Autodesk Inventor part; units mm, degrees
ref_plane "YZ Plane" through (0, 0, 0) normal (1, 0, 0) x (0, 1, 0)
ref_plane "XZ Plane" through (0, 0, 0) normal (0, 1, 0) x (-1, 0, 0)
ref_plane "XY Plane" through (0, 0, 0) normal (0, 0, 1) x (1, 0, 0)
sketch "Sketch1" plane through (0, 0, 0) normal (0, 1, 0) x (-1, 0, 0)
  line L0 (65, 81) -> (-65, 81)
  line L1 (-65, 81) -> (-65, -81)
  line L2 (-65, -81) -> (65, -81)
  line L3 (65, -81) -> (65, 81)
  point P0 (0, 0)
  point P1 (65, 0)
  point P2 (0, -81)
  dimension "d0" = 162
  dimension "d1" = 130
extrude "Extrusion1" add sketch "Sketch1" along normal blind 4
sketch "Sketch2" plane through (0, 4, 0) normal (0, 1, 0) x (1, 0, 0)
  circle A0 centre (-30, 0) radius 6
  circle A1 centre (30, 0) radius 6
  line L0 (-30, 6) -> (30, 6)
  line L1 (-30, -6) -> (30, -6)
  point P0 (0, 0)
  dimension "d4" = 12
  dimension "d5" = 12
  dimension "d6" = 30
  dimension "d7" = 30
extrude "Extrusion2" cut sketch "Sketch2" against normal through all
sketch "Sketch3" plane through (65, 0, 81) normal (1, 0, 0) x (0, 0, -1)
  line L0 (0, 4) -> (162, 4)
  line L1 (0, 0) -> (162, 0)
  line L2 (51, 4) -> (111, 4)
  line L3 (111, 4) -> (111, 0)
  line L4 (111, 0) -> (51, 0)
  line L5 (51, 0) -> (51, 4)
  point P0 (81, 0)
  point P1 (81, 0)
  dimension "d10" = 60
  dimension "d11" = 30
extrude "Extrusion3" add sketch "Sketch3" along normal blind 12
sketch "Sketch4" plane through (0, 4, 0) normal (0, 1, 0) x (1, 0, 0)
  line L0 (-65, -81) -> (65, -81)
  line L1 (-65, -81) -> (-55, -81)
  line L2 (-55, -81) -> (-55, -61)
  line L3 (-55, -61) -> (-65, -61)
  line L4 (-65, -61) -> (-65, -81)
  point P0 (0, 0)
  dimension "d14" = 20
  dimension "d15" = 10
extrude "Extrusion4" cut sketch "Sketch4" against normal blind 4
mirror "Mirror1" about plane through (0, 0, 0) normal (0, 0, 1) of "Extrusion4"
sketch "Sketch5" plane through (65, 0, 81) normal (0, 0, 1) x (1, 0, 0)
  line L0 (-35, 4) -> (-95, 4)
  line L1 (-80, 4) -> (-30, 4)
  line L2 (-30, 4) -> (-30, 0)
  line L3 (-30, 0) -> (-80, 0)
  line L4 (-80, 0) -> (-80, 4)
  line L5 (0, 0) -> (0, 4)
  point P0 (-65, 0)
  point P1 (-30, 2)
  point P2 (-80, 2)
  point P3 (0, 2)
  point P4 (-55, 0)
  dimension "d18" = 50
  dimension "d19" = 55
extrude "Extrusion5" add sketch "Sketch5" along normal blind 12
sketch "Sketch6" plane through (0, 4, 0) normal (0, 1, 0) x (1, 0, 0)
  line L0 (0, -85) -> (20, -85)
  line L1 (20, -85) -> (20, -89)
  line L2 (20, -89) -> (0, -89)
  line L3 (0, -89) -> (0, -85)
  line L4 (35, -81) -> (65, -81)
  line L5 (35, -81) -> (35, -93)
  point P0 (0, 0)
  point P1 (20, -87)
  dimension "d22" = 20
  dimension "d23" = 4
  dimension "d24" = 4
  dimension "d25" = 15
extrude "Extrusion6" cut sketch "Sketch6" against normal blind 12
mirror "Mirror2" about plane through (0, 0, 0) normal (0, 0, 1) of "Extrusion5", "Extrusion6"
sketch "Sketch7" plane through (0, 4, 0) normal (0, 1, 0) x (1, 0, 0)
  line L0 (69, 15) -> (73, 15)
  line L1 (73, 15) -> (73, -15)
  line L2 (73, -15) -> (69, -15)
  line L3 (69, -15) -> (69, 15)
  line L4 (65, 30) -> (65, 81)
  point P0 (0, 0)
  point P1 (69, 0)
  dimension "d28" = 4
  dimension "d29" = 4
  dimension "d30" = 30
extrude "Extrusion7" cut sketch "Sketch7" against normal blind 12
properties part number "Parte intermedia"
The model under review builds one solid part; all positions refer to its coordinate system, in mm. A direction names the side the tool comes from. Give positions to 0.01 mm unless a question says otherwise; leave off trailing zeros. Write each loop counter-clockwise with the first axis right and the second up, starting at its lowest first coordinate (ties: lowest second). Pieces come first, ordered by that corner, then holes. Notation, with made-up numbers: M 68.5,68.25 L 112.5,68.25 A17 cw 112.5,99.25 Z; hole C -20.75,-24.5 d3. An arc over 180 degrees is marked long. Write each question's results on one line, items separated by ' | '. Start each with the question number.
1. For probe 1 along Z at (x, y) = (1, 0.3); probe 2 along Z at (x, y) = (27, 3.3); probe 3 along X at (y, z) = (3.05, -10), list the stretches that pass through material, from the lowest coordinate up. Write a range as [from, to].
2. We need section D-D (z = 56). Write out the cut boundary in (x, y), and give its area (3 significant figures).
3. We need section B-B (x = -32). Write out the cut boundary in (y, z).
4. Insertion check: pin 1 Ø1.2 at (y, z) = (2, -86.5) entering from +X; pin 2 Ø3 at (x, z) = (-20.5, 11.5) entering from -Y; pin 3 Ø1 at (x, y) = (61.5, 2) entering from -Z. Each pin has a flat end and moves straight along its axis. Give the tip position at first contact, or say it passes through.
5. We need section C-C (y = 2.25). Count the separate pieces of the cut face and the enclosed holes in it, and give its area (3 significant figures).
6. For faces 1 (the flat face through (35, 2, 87)), 2 (the flat face through (-60, 2, 61)), 3 (the flat face through (35, 2, -87)), 4 (the flat face through (0, 2, -87)), 5 (the flat face through (77, 2, 0)), list the 3-axis set-ups (+Z, -Z, +X, -X, +Y, -Y) from which the entire face can be reached by the end or side of a thin tool; tool diameter is ignored.
7. We need section A-A (z = 2.5). Write out the cut boundary in (x, y).
Results found:
1) probe 1: z = [-93, -89], [-85, -6], [6, 85], [89, 93] | probe 2: z = [-93, -6], [6, 93] | probe 3: x = [-65, 69], [73, 77]
2) outline: M -65,0 L 65,0 L 65,4 L -65,4 Z | area: 520 mm^2
3) outline: M 0,-81 L 4,-81 L 4,-5.66 L 0,-5.66 Z; M 0,5.66 L 4,5.66 L 4,81 L 0,81 Z
4) pin 1: stops at x = 35 | pin 2: stops at y = 0 | pin 3: stops at z = -81
5) separate pieces: 1 | enclosed holes: 4 | area: 21,500 mm^2
6) face 1: +Z, +X, +Y, -Y | face 2: +Z, -X, +Y, -Y | face 3: -Z, +X, +Y, -Y | face 4: +Y, -Y | face 5: +Z, -Z, +X, +Y, -Y
7) outline: M -65,0 L -35.45,0 L -35.45,4 L -65,4 Z; M 35.45,0 L 69,0 L 69,4 L 35.45,4 Z; M 73,0 L 77,0 L 77,4 L 73,4 Z
